Autodesk Inventor part; units mm, degrees
ref_plane "YZ Plane" through (0, 0, 0) normal (1, 0, 0) x (0, 1, 0)
ref_plane "XZ Plane" through (0, 0, 0) normal (0, 1, 0) x (-1, 0, 0)
ref_plane "XY Plane" through (0, 0, 0) normal (0, 0, 1) x (1, 0, 0)
sketch "Sketch1" plane through (0, 0, 0) normal (0, 1, 0) x (-1, 0, 0)
  line L0 (0, 0) -> (6, 0)
  line L1 (6, 0) -> (6, -25)
  line L2 (6, -25) -> (0, -25)
  line L3 (0, -25) -> (0, 0)
  line L4 (0, -21) -> (0, -4)
  dimension "d0" = 25
  dimension "d1" = 6
sketch "Sketch2" plane through (0, 0, 0) normal (0, 0, 1) x (1, 0, 0)
  line L0 (0, 0) -> (-6, 0)
  line L1 (-6, 0) -> (-6, 10)
  line L2 (-6, 10) -> (0, 10)
  line L3 (0, 10) -> (0, 0)
  line L4 (0, 0) -> (-6, 3.5)
  line L5 (0, 10) -> (-6, 6.5)
  dimension "d5" = 10
  dimension "d6" = 6
  dimension "d13" = 3.5
  dimension "d14" = 3.5
sketch "Sketch3" plane through (0, 0, 0) normal (0, 1, 0) x (-1, 0, 0)
  line L0 (0, -4) -> (3, -4)
  line L1 (3, -4) -> (3, -21)
  line L2 (3, -21) -> (0, -21)
  line L3 (0, -21) -> (0, -4)
  point P0 (0, 0)
  dimension "d7" = 4
  dimension "d8" = 3
  dimension "d9" = 21
  dimension "d10" = 0
extrude "Extrusion1" add sketch "Sketch1" along normal blind 10
extrude "Extrusion2" cut sketch "Sketch3" along normal blind 10
extrude "Extrusion3" cut sketch "Sketch2" against normal blind 25 contours L5 L1 L2
extrude "Extrusion4" cut sketch "Sketch2" against normal blind 25 contours L0 L1 L4
equation "\"d6\" = d1"
equation "\"d13\" = d14"
equation "\"d11\" = d5"
equation "\"d15\" = d5"
equation "\"d17\" = d0"
equation "\"d19\" = d0"
properties part number "cable_tie_bracket"
Source: CAD feature listing. Evaluate the final solid. Frame: model axes, mm. A direction names the side the tool comes from. Coordinates: 2 decimals unless noted, no trailing zeros. Loops run counter-clockwise (first coordinate to the right, second up) from the corner with the lowest first, then second, coordinate; pieces in that order, holes last. Notation, with made-up numbers: M -30.75,-24 L -26.75,-24 A21 cw -26.75,-7 Z; hole C 31,-29.75 d5. An arc over 180 degrees is marked long. Answer in a Markdown table with one row per item.
Q1. Section A-A on x = -0.75. Return the cut outline in (y, z).
Answers below:
| item | result |
|---|---|
| outline | M 0.44,-25 L 9.56,-25 L 9.56,-21 L 0.44,-21 Z; M 0.44,-4 L 9.56,-4 L 9.56,0 L 0.44,0 Z |
Q2. First-contact query: pin 1 (4 mm diameter, centred on y = 6, z = -11.5, fed in from +X). Flat tip, straight axial feed; report the tip coordinate or a pass-through.
Answers below:
| item | result |
|---|---|
| pin 1 | stops at x = -3 |
Q3. Ray query, probe 1 along Z at (x, y) = (-2.75, 7.75); probe 2 along X at (y, z) = (5.25, -17.75); probe 3 along Y at (x, z) = (-3, -22). Return the intervals inside material, ascending. Write a range as from..to.
Answers below:
| item | result |
|---|---|
| probe 1 | z = -25..-21, -4..0 |
| probe 2 | x = -6..-3 |
| probe 3 | y = 1.75..8.25 |
Q4. Section B-B on y = 1.25. Return the cut outline in (x, z).
Answers below:
| item | result |
|---|---|
| outline | M -2.14,-25 L 0,-25 L 0,-21 L -2.14,-21 Z; M -2.14,-4 L 0,-4 L 0,0 L -2.14,0 Z |
Q5. Section C-C on y = 3.75. Return the cut outline in (x, z).
Answers below:
| item | result |
|---|---|
| outline | M -6,-25 L 0,-25 L 0,-21 L -3,-21 L -3,-4 L 0,-4 L 0,0 L -6,0 Z |
Q6. Set-up query: faces 4 (the flat face through (-3.6, 7.9, -12.3)), 5 (the flat face through (-2, 5, -21)). Return all of +Z, -Z, +X, -X, +Y, -Y with unobstructed straight access to the full face (end or side cutting, diameter ignored); none if empty.
Answers below:
| item | result |
|---|---|
| face 4 | +Z, -Z, -X, +Y |
| face 5 | +X, +Y, -Y |
Q7. Section D-D on z = -21.25. Return the cut outline in (x, y), plus the area to 3 significant figures.
Answers below:
| item | result |
|---|---|
| outline | M -6,3.5 L 0,0 L 0,10 L -6,6.5 Z |
| area | 39.0 mm^2 |
Q8. Draft query along Z for faces 1 (the flat face through (0, 5, -2)), 2 (the flat face through (-2, 5, 0)), 3 (the flat face through (-3, 5, -12)). Return one class per face: pulls with the +Z half, pulls with the -Z half, needs draft (parallel to the pull), parting line crosses it, or undercut.
Answers below:
| item | result |
|---|---|
| face 1 | needs draft |
| face 2 | pulls with the +Z half |
| face 3 | undercut |
